The drawing under review shows one solid part. Ordinate dimensions are in mm from its lowest x, y, z. Give positions to 0.01 mm unless a question says otherwise; leave off trailing zeros. Loops run counter-clockwise (first coordinate to the right, second up) from the corner with the lowest first, then second, coordinate; pieces in that order, holes last. Notation, with made-up numbers: M 63,21.25 L 67,21.25 A10 cw 67,40.25 Z; hole C 68,18.25 d2. An arc over 180 degrees is marked long. Put each result on its own line as item: value. Start each with the question number.
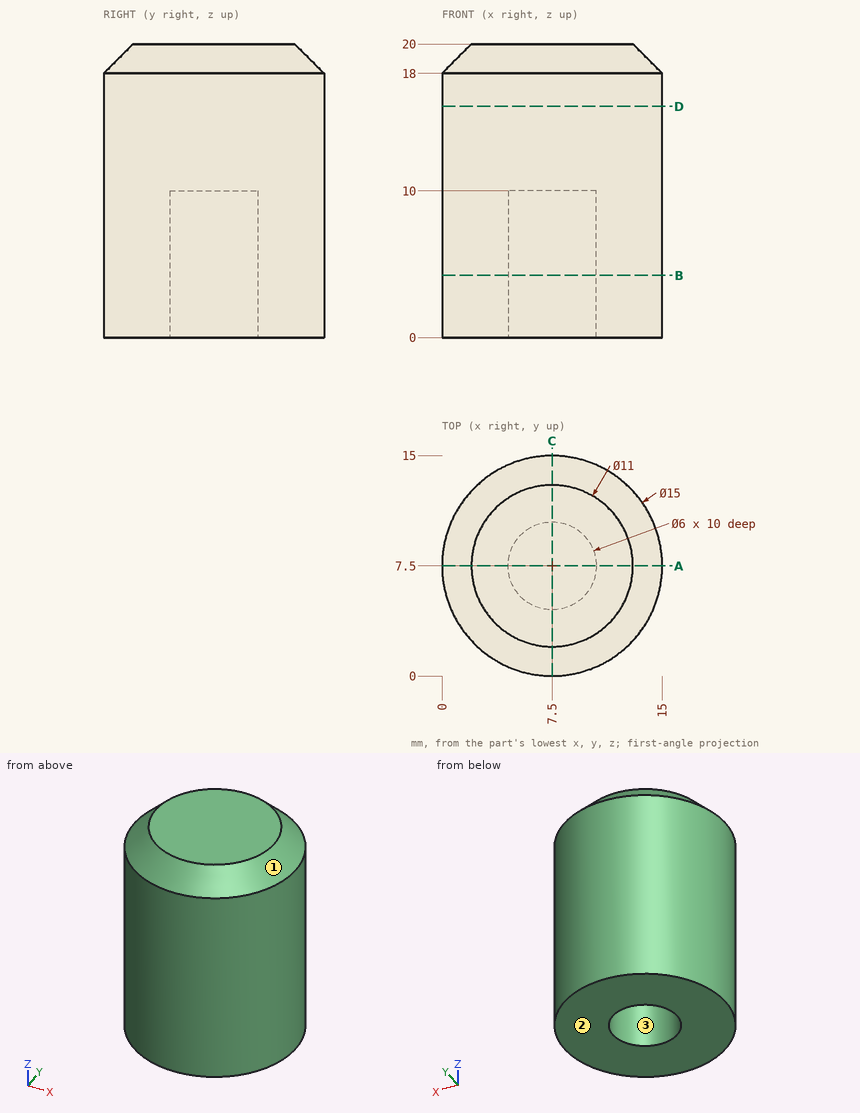
(1) To check wall thickness, follow L1, parallel to Y at x = 7.5, z = 3.75; L2, parallel to Z at x = 8.75, y = 9; L3, parallel to X at y = 4.75, z = 1.5. State the ranges of each line that lie inside material, in increasing order. Write a range as [from, to].
(2) Draft analysis for pull direction X (two halves, no side actions). For the marked faces 1, 2 and 3, state which applies: +X half, -X half, draft (parallel to the pull), parting line (faces both ways), or undercut.
(3) We need section B-B, the plane z = 4.25. Write out the cut boundary in (x, y).
(4) We need section D-D, the plane z = 15.75. Write out the cut boundary in (x, y).
(5) We need section A-A, the plane y = 7.5. Write out the cut boundary in (x, z).
(6) Insertion check: pin 1 (4 mm diameter, centred on y = 1.5, z = 17.5, fed in from -X); pin 2 (3 mm diameter, centred on y = 10, z = 13, fed in from +X); pin 3 (5 mm diameter, centred on y = 3.5, z = 17, fed in from +X). Each pin has a flat end and moves straight along its axis. Give the tip position at first contact, or say it passes through.
Check sheet entries:
1. L1: y = [0, 4.5], [10.5, 15]
1. L2: z = [10, 20]
1. L3: x = [0.52, 6.3], [8.7, 14.48]
2. face 1: parting line
2. face 2: draft
2. face 3: undercut
3. outline: C 7.5,7.5 d15; hole C 7.5,7.5 d6
4. outline: C 7.5,7.5 d15
5. outline: M 0,0 L 4.5,0 L 4.5,10 L 10.5,10 L 10.5,0 L 15,0 L 15,18 L 13,20 L 2,20 L 0,18 Z
6. pin 1: stops at x = 1.16
6. pin 2: stops at x = 14.93
6. pin 3: stops at x = 14.85
